Input: part model. Units: mm. Frame: model coordinates. A direction names the side the tool comes from. Give positions to 0.01 mm unless a question says otherwise; leave off trailing zeros. Loops run counter-clockwise (first coordinate to the right, second up) from the corner with the lowest first, then second, coordinate; pieces in that order, holes last. Notation, with made-up numbers: M 82.25,1 L 138.25,1 A30 ccw 138.25,39 Z; hole C 21.5,-23 d10. An arc over 180 degrees is marked long. Answer as a JSON object with one key per item and string values. Group by question number.
1) Ray query, L1, parallel to X at y = 15.35, z = -5; L2, parallel to X at y = 6.25, z = 1.25; L3, parallel to Y at x = -3.5, z = -3.75. Return the intervals inside material, ascending.
2) Draft query along X for faces 6 (the cylindrical face through (19.086, 15.021, 4.792)), 7 (the flat face through (0, 1, -8.5)), 8 (the cylindrical face through (11.86, 12.6, -0.12)). Return one class per face: +X half, -X half, draft (parallel to the pull), parting line (faces both ways), or undercut.
3) Section query B-B on x = 17.5. Return loops of the section in (y, z), plus the area to 3 significant figures.
4) Section query D-D on y = 5.75. Return loops of the section in (x, z), plus the area to 3 significant figures.
5) Section query A-A on y = 15.25. Return loops of the section in (x, z).
6) First-contact query: P1, Ø5, axis at y = 3.5, z = -0.5, coming from the +X side; P2, Ø4, axis at x = 17.5, z = -5, coming from the -Y side; P3, Ø1.9, axis at x = -17.5, z = 5, coming from the -Y side; P4, Ø5, axis at x = 0, z = 0, coming from the +Y side. Flat tips, straight axial feed; report the tip coordinate or a pass-through.
7) Access query for faces 1 (the flat face through (15, 16.5, 0)), 2 (the flat face through (0, 0, 0)), 3 (the flat face through (0, 3, 0)), 4 (the flat face through (-11, 5, 0)), 5 (the flat face through (17, 13.5, 0)). Directions: +Z, -Z, +X, -X, +Y, -Y. A direction counts if a zero-diameter tool reaches every point of the face in a straight line with its end or side. Return the directions, or none.
8) Section query C-C on z = -5. Return loops of the section in (x, y).
from build123d import *

# Parameters (mm, degrees)
SKETCH_1_W          = 22
SKETCH_1_H          = 17
EXTRUDE_1_DEPTH     = 3
SKETCH_2_W          = 2.75
SKETCH_2_H          = 17
EXTRUDE_2_DEPTH     = 13.5
SKETCH_3_W          = 10
SKETCH_3_H          = 17
EXTRUDE_3_DEPTH     = 3
CUT_EXTRUDE_1_REACH = 30.027
SKETCH_4_R          = 1.6
FILLET_1_R          = 3


with BuildPart() as part:
    # 草图1 → 凸台-拉伸1 (new body)
    with BuildSketch(Plane(origin=(0, 0, 0), x_dir=(1, 0, 0), z_dir=(0, 1, 0))):
        Rectangle(SKETCH_1_W, SKETCH_1_H)
    extrude(amount=EXTRUDE_1_DEPTH)

    # 草图2 → 凸台-拉伸2 (add)
    with BuildSketch(Plane(origin=(0, 3, 0), x_dir=(1, 0, 0), z_dir=(0, 1, 0))):
        with Locations((-9.625, 0)):
            Rectangle(SKETCH_2_W, SKETCH_2_H)
        with Locations((9.625, 0)):
            Rectangle(SKETCH_2_W, SKETCH_2_H)
    extrude(amount=EXTRUDE_2_DEPTH)

    # 草图3 → 凸台-拉伸3 (add)
    with BuildSketch(Plane(origin=(0, 16.5, 0), x_dir=(1, 0, 0), z_dir=(0, 1, 0))):
        with Locations((16, 0)):
            Rectangle(SKETCH_3_W, SKETCH_3_H)
        with Locations((-16, 0)):
            Rectangle(SKETCH_3_W, SKETCH_3_H)
    extrude(amount=-EXTRUDE_3_DEPTH)

    # 草图4 → 切除-拉伸1 (cut, up to next)
    with BuildSketch(Plane(origin=(0, 16.5, 0), x_dir=(1, 0, 0), z_dir=(0, 1, 0)), mode=Mode.PRIVATE) as cut_extrude_1_sk1:
        with Locations(Location((-17.5, 5, 0), (0, 0, 270))):
            Circle(SKETCH_4_R)
    cut_extrude_1_tool1 = extrude(cut_extrude_1_sk1.sketch, amount=-CUT_EXTRUDE_1_REACH, mode=Mode.PRIVATE) & part.part
    # 草图4 → 切除-拉伸1 (cut, up to next)
    with BuildSketch(Plane(origin=(0, 16.5, 0), x_dir=(1, 0, 0), z_dir=(0, 1, 0)), mode=Mode.PRIVATE) as cut_extrude_1_sk2:
        with Locations(Location((-17.5, -5, 0), (0, 0, 90))):
            Circle(SKETCH_4_R)
    cut_extrude_1_tool2 = extrude(cut_extrude_1_sk2.sketch, amount=-CUT_EXTRUDE_1_REACH, mode=Mode.PRIVATE) & part.part
    # 草图4 → 切除-拉伸1 (cut, up to next)
    with BuildSketch(Plane(origin=(0, 16.5, 0), x_dir=(1, 0, 0), z_dir=(0, 1, 0)), mode=Mode.PRIVATE) as cut_extrude_1_sk3:
        with Locations(Location((17.5, -5, 0), (0, 0, 270))):
            Circle(SKETCH_4_R)
    cut_extrude_1_tool3 = extrude(cut_extrude_1_sk3.sketch, amount=-CUT_EXTRUDE_1_REACH, mode=Mode.PRIVATE) & part.part
    # 草图4 → 切除-拉伸1 (cut, up to next)
    with BuildSketch(Plane(origin=(0, 16.5, 0), x_dir=(1, 0, 0), z_dir=(0, 1, 0)), mode=Mode.PRIVATE) as cut_extrude_1_sk4:
        with Locations(Location((17.5, 5, 0), (0, 0, 270))):
            Circle(SKETCH_4_R)
    cut_extrude_1_tool4 = extrude(cut_extrude_1_sk4.sketch, amount=-CUT_EXTRUDE_1_REACH, mode=Mode.PRIVATE) & part.part
    add(cut_extrude_1_tool1.solids().sort_by_distance((-17.5, 16.5, -5))[0], mode=Mode.SUBTRACT)
    add(cut_extrude_1_tool2.solids().sort_by_distance((-17.5, 16.5, 5))[0], mode=Mode.SUBTRACT)
    add(cut_extrude_1_tool3.solids().sort_by_distance((17.5, 16.5, 5))[0], mode=Mode.SUBTRACT)
    add(cut_extrude_1_tool4.solids().sort_by_distance((17.5, 16.5, -5))[0], mode=Mode.SUBTRACT)

    # 圆角1
    fillet_1_edges = [part.edges().sort_by_distance(p)[0] for p in [
        (11, 13.5, 0),
        (-11, 13.5, 0),
    ]]
    fillet(fillet_1_edges, radius=FILLET_1_R)


solid = part.part
Output:
{
 "1": {"L1": "x = -21 to -19.1, -15.9 to -8.25, 8.25 to 15.9, 19.1 to 21", "L2": "x = -11 to -8.25, 8.25 to 11", "L3": "y = 0 to 3"},
 "2": {"face 6": "undercut", "face 7": "draft", "face 8": "+X half"},
 "3": {"outline": "M 13.5,-8.5 L 16.5,-8.5 L 16.5,-6.6 L 13.5,-6.6 Z; M 13.5,-3.4 L 16.5,-3.4 L 16.5,3.4 L 13.5,3.4 Z; M 13.5,6.6 L 16.5,6.6 L 16.5,8.5 L 13.5,8.5 Z", "area": "31.8 mm^2"},
 "4": {"outline": "M -11,-8.5 L -8.25,-8.5 L -8.25,8.5 L -11,8.5 Z; M 8.25,-8.5 L 11,-8.5 L 11,8.5 L 8.25,8.5 Z", "area": "93.5 mm^2"},
 "5": {"outline": "M -21,-8.5 L -8.25,-8.5 L -8.25,8.5 L -21,8.5 Z; M 8.25,-8.5 L 21,-8.5 L 21,8.5 L 8.25,8.5 Z; hole C -17.5,-5 d3.2; hole C -17.5,5 d3.2; hole C 17.5,-5 d3.2; hole C 17.5,5 d3.2"},
 "6": {"P1": "stops at x = 11", "P2": "stops at y = 13.5", "P3": "passes through", "P4": "stops at y = 3"},
 "7": {"face 1": "+Z, -Z, +X, -X, +Y", "face 2": "+Z, -Z, +X, -X, -Y", "face 3": "+Z, -Z, +Y", "face 4": "+Z, -Z, -X, -Y", "face 5": "+Z, -Z, +X, -Y"},
 "8": {"outline": "M -21,13.5 L -19.1,13.5 L -19.1,16.5 L -21,16.5 Z; M -15.9,13.5 L -14,13.5 A3 cw -11,10.5 L -11,0 L 11,0 L 11,10.5 A3 cw 14,13.5 L 15.9,13.5 L 15.9,16.5 L 8.25,16.5 L 8.25,3 L -8.25,3 L -8.25,16.5 L -15.9,16.5 Z; M 19.1,13.5 L 21,13.5 L 21,16.5 L 19.1,16.5 Z"}
}
